Part model, mm, in its own coordinate system. Coordinates: 2 decimals unless noted, no trailing zeros. Write each loop counter-clockwise with the first axis right and the second up, starting at its lowest first coordinate (ties: lowest second). Pieces come first, ordered by that corner, then holes. Notation, with made-up numbers: (25, 78) -> (59, 78) arc R16 ccw to (59, 90) -> close; hole circle Ø2 at (-25.5, 53). An arc over 180 degrees is marked (long way). Write item = value, one per line. Start each with the question number.
Q1. Pin check, flat tip, straight feed: P1, Ø2.5, axis at x = 0, y = -28.575, coming from the +Z side. Stop position of the tip, or through.
Q2. Pull direction Y, two halves, no side cores. Call faces 1 (the flat face through (0, -31.75, 3)), 2 (the cylindrical face through (0.879, -30.265, 3.131)), 3 (the flat face through (0, 38.1, 3)), 4 (the flat face through (-25.4, 4, 3)): released by +Y, released by -Y, zero draft, split by the parting line, or undercut.
Q3. Band-saw the part on A-A, the plane x = 0. List the corners of the cut face in (y, z) (3 decimals).
Q4. Probe line 1 (Y direction, x = 0, z = 1.5) (3 decimals); line 2 (Y direction, x = 0.5, z = 3.5); line 3 (X direction, y = -29, z = 2.75). List the from-to ranges inside material, lowest first.
from build123d import *

# Parameters (mm, degrees)
F0_W     = 50.8
F0_H     = 50.8
F0_R     = 1.905
F0_H_2   = 6.35
F1_DEPTH = 6.35


with BuildPart() as f1:
    # F0 (on Top) → F1 (new body)
    with BuildSketch(Plane.XY):
        Rectangle(F0_W, F0_H)
        Polygon((-25.4, 31.750001), (-25.4, 25.4), (25.4, 25.4), (25.4, 31.750001), (25.4, 38.100001), (14.365858, 38.100001), (-14.365858, 38.100001), (-25.4, 38.100001), align=None)
        with Locations((0, 31.750001)):
            Circle(F0_R, mode=Mode.SUBTRACT)
        with Locations((0, -28.575)):
            Rectangle(F0_W, F0_H_2)
        with Locations((0, -28.575)):
            Circle(F0_R, mode=Mode.SUBTRACT)
    extrude(amount=F1_DEPTH)


solid = f1.part
Ans:
q1.P1 = through
q2.face_1 = released by -Y
q2.face_2 = undercut
q2.face_3 = released by +Y
q2.face_4 = zero draft
q3.outline = (-31.75, 0) -> (-30.48, 0) -> (-30.48, 6.35) -> (-31.75, 6.35) -> close; (-26.67, 0) -> (29.845, 0) -> (29.845, 6.35) -> (-26.67, 6.35) -> close; (33.655, 0) -> (38.1, 0) -> (38.1, 6.35) -> (33.655, 6.35) -> close
q4.line_1 = -31.75 to -30.48, -26.67 to 29.845, 33.655 to 38.1
q4.line_2 = -31.75 to -30.41, -26.74 to 29.91, 33.59 to 38.1
q4.line_3 = -25.4 to -1.86, 1.86 to 25.4
